The model under review builds one solid part; all positions refer to its coordinate system, in mm. A direction names the side the tool comes from. Coordinates: 2 decimals unless noted, no trailing zeros. Order: outer loops, then holes, each group sorted by start corner. A loop starts at its lowest first (then second) coordinate and runs counter-clockwise, first axis right, second up. Notation, with made-up numbers: (34, 44) -> (54, 44) arc R25 ccw to (54, 80) -> close; hole circle Ø10 at (11.5, -28). An arc over 180 degrees is marked (long way). Use CSV: the item, a comma, the result in double quotes. Start each with the question number.
Autodesk Inventor part; units mm, degrees
ref_plane "YZ Plane" through (0, 0, 0) normal (1, 0, 0) x (0, 1, 0)
ref_plane "XZ Plane" through (0, 0, 0) normal (0, 1, 0) x (-1, 0, 0)
ref_plane "XY Plane" through (0, 0, 0) normal (0, 0, 1) x (1, 0, 0)
sketch "Sketch1" plane through (0, 0, 0) normal (0, 1, 0) x (-1, 0, 0)
  circle A0 centre (0, 0) radius 18.542 construction
  circle A1 centre (0, 0) radius 24.892
  dimension "d0" = 37.084
  dimension "d1" = 6.35
extrude "Extrusion1" add sketch "Sketch1" along normal blind 11.43
sketch "Sketch2" plane through (0, 11.43, 0) normal (0, 1, 0) x (1, 0, 0)
  circle A0 centre (0, 0) radius 18.669
  dimension "d4" = 37.338
extrude "Extrusion2" cut sketch "Sketch2" against normal blind 7.62
sketch "Sketch3" plane through (0, 0, 0) normal (0, -1, 0) x (1, 0, 0)
  circle A0 centre (0, 0) radius 22.1615
  circle A1 centre (0, 0) radius 9.779
  dimension "d7" = 44.323
  dimension "d10" = 19.558
extrude "Extrusion4" cut sketch "Sketch3" against normal blind 2.7178
sketch "Sketch4" plane through (0, 0, 0) normal (0, -1, 0) x (1, 0, 0)
  line L0 (31.242, -6.35) -> (18.542, -6.35)
  line L1 (18.542, -6.35) -> (18.542, 6.35)
  line L2 (18.542, 6.35) -> (31.242, 6.35)
  line L3 (31.242, 6.35) -> (31.242, -6.35)
  circle A0 centre (0, 0) radius 24.892
  line L4 (31.242, -6.35) -> (18.542, 6.35) construction
  line L5 (18.542, -6.35) -> (31.242, 6.35) construction
  point P0 (24.892, 0)
  dimension "d13" = 12.7
  dimension "d14" = 12.7
extrude "Extrusion5" cut sketch "Sketch4" against normal up to surface (2.7178 mm away) contours L0 A0 L2 L3 | L0 L1 L2 A0 picked at (20.6587, 0)
properties part number "Lower Power"
Q1. Add section B-B, the plane x = 0. State the section outline as (y, z) points, then the cut area to 3 significant figures.
Q2. Add section C-C, the plane z = 0. State the section outline as (x, y) points.
Q3. Add section A-A, the plane y = 1.75. State the section outline as (x, z) points.
Q4. For faces 5 (the flat face through (23, 1, -6.35)), 6 (the flat face through (-4, 11.43, 19)), 7 (the cylindrical face through (-2.12, 1.34, -9.546)), 8 (the cylindrical face through (17.807, 7.673, -5.608)), list the 3-axis set-ups (+Z, -Z, +X, -X, +Y, -Y) from which the entire face can be reached by the end or side of a thin tool; tool diameter is ignored.
Q5. To check wall thickness, follow probe 1 along Z at (x, y) = (0, 2); probe 2 along Y at (x, z) = (14.5, -4.5); probe 3 along Y at (x, z) = (-1.5, 22). State the ranges of each line that lie inside material, in increasing order.
Q6. Clearance check with flat-ended pins moving along their axes: pin 1 Ø6 at (x, y) = (6.5, 8.5) entering from -Z; pin 2 Ø4 at (y, z) = (2, -3.5) entering from +X; pin 3 Ø2 at (x, y) = (-17, 9.5) entering from -Z. State where each tip first meets the part, or that it passes through.
Q7. Draft analysis for pull direction X (two halves, no side actions). For faces 1 (the cylindrical face through (-22.994, 5.635, 9.534)), 2 (the cylindrical face through (-22.144, 1.34, 0.884)), 3 (the flat face through (23, 1, 6.35)), 4 (the flat face through (0, 3.81, 0)), state which applies: +X half, -X half, draft (parallel to the pull), parting line (faces both ways), or undercut.
Q8. Add section D-D, the plane y = 10.75. State the section outline as (x, z) points.
Answer block:
1,outline,"(0, -24.89) -> (11.43, -24.89) -> (11.43, -18.67) -> (3.81, -18.67) -> (3.81, 18.67) -> (11.43, 18.67) -> (11.43, 24.89) -> (0, 24.89) -> (0, 22.16) -> (2.72, 22.16) -> (2.72, 9.78) -> (0, 9.78) -> (0, -9.78) -> (2.72, -9.78) -> (2.72, -22.16) -> (0, -22.16) -> close"
1,area,"217 mm²"
2,outline,"(-24.89, 0) -> (-22.16, 0) -> (-22.16, 2.72) -> (-9.78, 2.72) -> (-9.78, 0) -> (9.78, 0) -> (9.78, 2.72) -> (24.89, 2.72) -> (24.89, 11.43) -> (18.67, 11.43) -> (18.67, 3.81) -> (-18.67, 3.81) -> (-18.67, 11.43) -> (-24.89, 11.43) -> close"
3,outline,"circle Ø19.56 at (0, 0); (21.23, -6.35) arc R22.16 cw (long way) to (21.23, 6.35) -> (24.07, 6.35) arc R24.89 ccw (long way) to (24.07, -6.35) -> close"
4,face 5,"+X, -Y"
4,face 6,"+Z, -Z, +X, -X, +Y"
4,face 7,"-Y"
4,face 8,"+Y"
5,probe 1,"z = -24.89 to -22.16, -9.78 to 9.78, 22.16 to 24.89"
5,probe 2,"y = 2.72 to 3.81"
5,probe 3,"y = 2.72 to 11.43"
6,pin 1,"stops at z = -24.64"
6,pin 2,"stops at x = 24.84"
6,pin 3,"stops at z = -19.07"
7,face 1,"parting line"
7,face 2,"undercut"
7,face 3,"draft"
7,face 4,"undercut"
8,outline,"circle Ø49.78 at (0, 0); hole circle Ø37.34 at (0, 0)"
